Work out the finished part from the listing and answer in its coordinate system (mm). Face numbers are marked on the shaded views. A direction names the side the tool comes from. Coordinates: 2 decimals unless noted, no trailing zeros. Write each loop counter-clockwise with the first axis right and the second up, starting at its lowest first coordinate (ties: lowest second). Pieces come first, ordered by that corner, then holes. Notation, with made-up numbers: (47.5, 27.5) - (74.5, 27.5) arc R7 cw to (74.5, 32.5) - close; hole circle Ø2 at (-31, 27.25). An arc over 180 degrees is marked (long way). One line per item, written item: value.
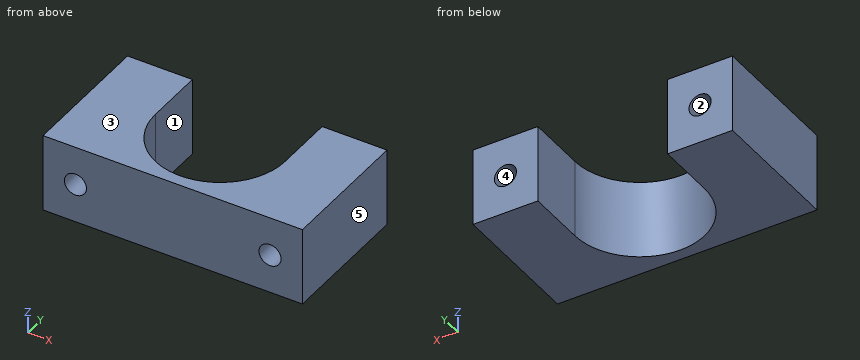
Solid Edge part; units mm, degrees
sketch "Sketch1" plane through (0, 0, 0) normal (0, 0, 1) x (1, 0, 0)
  line L0 (-10, 0) -> (-10, 9.2)
  line L1 (-10, 9.2) -> (-20, 9.2)
  line L2 (-20, 9.2) -> (-20, -11.8)
  line L3 (-20, -11.8) -> (20, -11.8)
  line L4 (20, -11.8) -> (20, 9.2)
  line L5 (20, 9.2) -> (10, 9.2)
  line L6 (10, 9.2) -> (10, 0)
  arc A0 (10, 0) -> (-10, 0) centre (0, 0) cw
  dimension "D1" = 10
  dimension "D2" = 20
  dimension "D3" = 20
extrude "Protrusion1" add sketch "Sketch1" along normal blind 20
sketch "Sketch2" plane through (-15, 9.2, 10) normal (0, 1, 0) x (0, 0, -1)
  circle A0 centre (4, -30) radius 1.7
  circle A1 centre (4, 0) radius 1.7
  dimension "D1" = 4
  dimension "D2" = 4
  dimension "D3" = 4
extrude "Cutout1" cut sketch "Sketch2" against normal through all
sketch "Sketch3" plane through (0, -11.8, 10) normal (0, -1, 0) x (1, 0, 0)
  line L0 (-20, 10) -> (-20, 2)
  line L1 (-20, 2) -> (20, 2)
  dimension "D1" = 20
extrude "Cutout2" cut sketch "Sketch3" against normal through all material side at (-19.95, -11.8, 16)
properties material "ABS Plastic, medium impact"
Item 1: Consider probe 1 along X at (y, z) = (3.75, 6); probe 2 along X at (y, z) = (4.5, 5); probe 3 along X at (y, z) = (5.75, 4.25). Determine where each line is inside the solid, lowest interval first.
Evaluation:
probe 1: x = -20 to -16.7, -13.3 to -10, 10 to 13.3, 16.7 to 20
probe 2: x = -20 to -16.37, -13.63 to -10, 10 to 13.63, 16.37 to 20
probe 3: x = -20 to -10, 10 to 20
Item 2: Given pin 1 (2 mm diameter, centred on x = -15, z = 6, fed in from -Y); pin 2 (1 mm diameter, centred on x = -10.5, y = -8.5, fed in from -Z); pin 3 (2 mm diameter, centred on x = -1, z = 10, fed in from +Y), each flat-ended and moving along its own axis, determine where each tip first touches the part or whether it passes through.
Evaluation:
pin 1: passes through
pin 2: stops at z = 0
pin 3: stops at y = -9.8
Item 3: Which of the six approach directions +Z, -Z, +X, -X, +Y, -Y give full straight-line access (tool end or side, diameter ignored) to the marked faces 1 and 2?
Evaluation:
face 1: +Z, -Z, +Y
face 2: +Y, -Y
Item 4: Determine the mould class of the marked faces 3, 4 and 5 for opening direction Z: +Z half, -Z half, draft (parallel to the pull), parting line (faces both ways), or undercut.
Evaluation:
face 3: +Z half
face 4: undercut
face 5: draft
Item 5: Section B-B, the plane y = 6.75 is taken. Determine the outline of the cut face in (x, z).
Evaluation:
outline: (-20, 0) - (-10, 0) - (-10, 12) - (-20, 12) - close; (10, 0) - (20, 0) - (20, 12) - (10, 12) - close; hole circle Ø3.4 at (-15, 6); hole circle Ø3.4 at (15, 6)
Item 6: Section C-C, the plane x = -15 is taken. Determine the outline of the cut face in (y, z).
Evaluation:
outline: (-11.8, 0) - (9.2, 0) - (9.2, 4.3) - (-11.8, 4.3) - close; (-11.8, 7.7) - (9.2, 7.7) - (9.2, 12) - (-11.8, 12) - close
Item 7: Section A-A, the plane z = 6 is taken. Determine the outline of the cut face in (x, y).
Evaluation:
outline: (-20, -11.8) - (-16.7, -11.8) - (-16.7, 9.2) - (-20, 9.2) - close; (-13.3, -11.8) - (13.3, -11.8) - (13.3, 9.2) - (10, 9.2) - (10, 0) arc R10 cw to (-10, 0) - (-10, 9.2) - (-13.3, 9.2) - close; (16.7, -11.8) - (20, -11.8) - (20, 9.2) - (16.7, 9.2) - close
Item 8: Section D-D, the plane z = 11.25 is taken. Determine the outline of the cut face in (x, y), then the cut area to 3 significant figures.
Evaluation:
outline: (-20, -11.8) - (20, -11.8) - (20, 9.2) - (10, 9.2) - (10, 0) arc R10 cw to (-10, 0) - (-10, 9.2) - (-20, 9.2) - close
area: 499 mm2
